Can you work these out from the drawing? Everything is in mm from the part's minimum corner. Give positions to 0.01 mm unless a question says otherwise; leave off trailing zeros. Write each loop counter-clockwise with the first axis right and the second up, starting at its lowest first coordinate (ties: lowest second). Pieces come first, ordered by that corner, then holes. Notation, with made-up numbers: (-14.75, -8) -> (-8.75, -8) arc R9 cw to (-8.75, 8) -> close; hole circle Ø11 at (15.25, 0). An arc over 180 degrees is marked (long way). Answer as CSV lines item,"result". Start each with the question number.
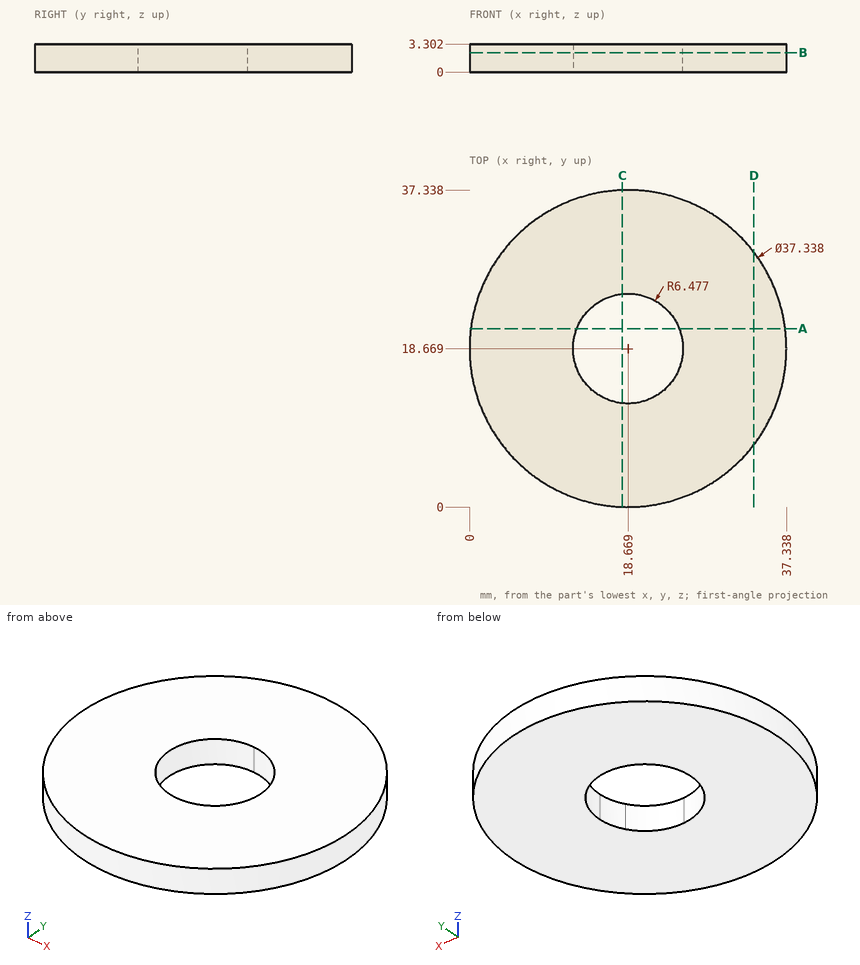
Item 1: If we section it at A-A (y = 21): Please give me the cut outline in (x, z).
Item 2: If we section it at B-B (z = 2.3): Please give me the cut outline in (x, y).
Item 3: I'm going to push flat-ended pins straight in: pin 1 (1 mm diameter, centred on y = 8.5, z = 0.5, fed in from +X); pin 2 (1.5 mm diameter, centred on x = 22, z = 1.5, fed in from +Y). Where does each tip first touch, or does it pass through?
Item 4: If we section it at D-D (x = 33.5): Please give me the cut outline in (y, z), and give its area (3 significant figures).
Item 5: If I drill on line 1 (Y direction, x = 17.5, z = 2.55); line 2 (Y direction, x = 19, z = 2.1); line 3 (X direction, y = 35, z = 0.55) (3 decimals), over which ranges is the centre line in solid material (lowest first)? Write a range as [from, to].
Item 6: If we section it at C-C (x = 18): Please give me the cut outline in (y, z).
Final values:
1,outline,"(0.15, 0) -> (12.63, 0) -> (12.63, 3.3) -> (0.15, 3.3) -> close; (24.71, 0) -> (37.19, 0) -> (37.19, 3.3) -> (24.71, 3.3) -> close"
2,outline,"circle Ø37.34 at (18.67, 18.67); hole circle Ø12.95 at (18.67, 18.67)"
3,pin 1,"x = 34.64"
3,pin 2,"y = 37.16"
4,outline,"(7.33, 0) -> (30.01, 0) -> (30.01, 3.3) -> (7.33, 3.3) -> close"
4,area,"74.9 mm2"
5,line 1,"[0.04, 12.3], [25.04, 37.3]"
5,line 2,"[0, 12.2], [25.14, 37.34]"
5,line 3,"[9.623, 27.715]"
6,outline,"(0.01, 0) -> (12.23, 0) -> (12.23, 3.3) -> (0.01, 3.3) -> close; (25.11, 0) -> (37.33, 0) -> (37.33, 3.3) -> (25.11, 3.3) -> close"
